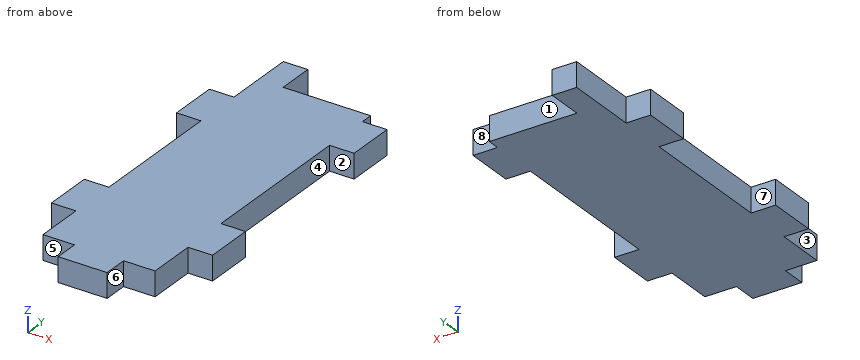
```python
from build123d import *

# Parameters (mm, degrees)
ESQUISSE1_W             = 32.86
ESQUISSE1_H             = 73
BOSS_EXTRU_1_DEPTH      = 5
ESQUISSE2_W             = 5
ESQUISSE2_H             = 33
ESQUISSE2_H_2           = 15
ESQUISSE2_H_3           = 10
ESQUISSE2_H_4           = 28
ENL_V_MAT_EXTRU_1_DEPTH = 5
ESQUISSE3_W             = 10
ESQUISSE3_H             = 5
BOSS_EXTRU_2_DEPTH      = 5


with BuildPart() as part:
    # Esquisse1 → Boss.-Extru.1 (new body)
    with BuildSketch(Plane.XY):
        with Locations((159.387093212, -0.522583191)):
            Rectangle(ESQUISSE1_W, ESQUISSE1_H)
    extrude(amount=BOSS_EXTRU_1_DEPTH)

    # Esquisse2 → Enlèv. mat.-Extru.1 (cut)
    with BuildSketch(Plane.XY.offset(5)):
        Polygon((170.817093212, 25.977416809), (170.817093212, 28.477416809), (152.957093212, 28.477416809), (152.957093212, 35.977416809), (175.817093212, 35.977416809), (175.817093212, 25.977416809), align=None)
        with Locations((173.317093212, -0.522583191)):
            Rectangle(ESQUISSE2_W, ESQUISSE2_H)
        with Locations((145.457093212, 28.477416809)):
            Rectangle(ESQUISSE2_W, ESQUISSE2_H_2)
        with Locations((173.317093212, -32.022583191)):
            Rectangle(ESQUISSE2_W, ESQUISSE2_H_3)
        with Locations((145.457093212, -32.022583191)):
            Rectangle(ESQUISSE2_W, ESQUISSE2_H_3)
        with Locations((145.457093212, -3.022583191)):
            Rectangle(ESQUISSE2_W, ESQUISSE2_H_4)
    extrude(amount=-ENL_V_MAT_EXTRU_1_DEPTH, mode=Mode.SUBTRACT)

    # Esquisse3 → Boss.-Extru.2 (add)
    with BuildSketch(Plane.XY.offset(5)):
        with Locations((159.387093212, -39.522583191)):
            Rectangle(ESQUISSE3_W, ESQUISSE3_H)
    extrude(amount=-BOSS_EXTRU_2_DEPTH)


solid = part.part
```
Model file for the job. Use its own axes, mm. Face numbers are marked on the shaded views. A direction names the side the tool comes from. Round coordinates to 2 decimals unless told otherwise and drop trailing zeros. Loops run counter-clockwise (first coordinate to the right, second up) from the corner with the lowest first, then second, coordinate; pieces in that order, holes last. Notation, with made-up numbers: M 24.25,-14.75 L 81.25,-14.75 A17 cw 81.25,17.25 Z; hole C 13,-39 d3. An arc over 180 degrees is marked long. Put each result on its own line as item: value. Start each with the question number.
Item 1: Cut at D-D (x = 166.5). List the corners of the cut face in (y, z).
Item 2: Drop flat-ended pins along their axis: P1, Ø1.5, axis at x = 144.5, z = 3.5, coming from the -Y side; P2, Ø2.5, axis at x = 174.5, z = 2, coming from the +Y side; P3, Ø8, axis at x = 165, y = 9.5, coming from the -Z side; P4, Ø1.5, axis at x = 146.5, z = 3.5, coming from the +Y side. Give the stop position or say it passes through.
Item 3: Cut at B-B (z = 1.3). List the corners of the cut face in (x, y).
Item 4: Cut at C-C (y = 12). List the corners of the cut face in (x, z), then the cut area to 3 significant figures.
Item 5: Mould opens along Y. For the marked faces 1, 2, 3 and 4 say: released by +Y, released by -Y, zero draft, split by the parting line, or undercut.
Item 6: Drill centre lines: line 1 along Y through (x, z) = (173.5, 2.6); line 2 along Y through (x, z) = (145.5, 0.6); line 3 along Y through (x, z) = (170, 2.65). Where is each one in solid material? Low to high.
Item 7: 3-axis set-ups, long thin cutter, end or side, ignore diameter. For the marked faces 5, 6, 7 and 8: which of +Z, -Z, +X, -X, +Y, -Y reach the whole face in a straight line?
Item 8: Cut at A-A (x = 147). List the corners of the cut face in (y, z).
Answer block:
1. outline: M -37.02,0 L 28.48,0 L 28.48,5 L -37.02,5 Z
2. P1: y = -27.02
2. P2: y = 25.98
2. P3: z = 0
2. P4: y = 20.98
3. outline: M 142.96,-27.02 L 147.96,-27.02 L 147.96,-37.02 L 154.39,-37.02 L 154.39,-42.02 L 164.39,-42.02 L 164.39,-37.02 L 170.82,-37.02 L 170.82,-27.02 L 175.82,-27.02 L 175.82,-17.02 L 170.82,-17.02 L 170.82,15.98 L 175.82,15.98 L 175.82,25.98 L 170.82,25.98 L 170.82,28.48 L 152.96,28.48 L 152.96,35.98 L 147.96,35.98 L 147.96,20.98 L 142.96,20.98 L 142.96,10.98 L 147.96,10.98 L 147.96,-17.02 L 142.96,-17.02 Z
4. outline: M 142.96,0 L 170.82,0 L 170.82,5 L 142.96,5 Z
4. area: 139 mm2
5. face 1: released by +Y
5. face 2: undercut
5. face 3: zero draft
5. face 4: undercut
6. line 1: -27.02 to -17.02, 15.98 to 25.98
6. line 2: -27.02 to -17.02, 10.98 to 20.98
6. line 3: -37.02 to 28.48
7. face 5: +Z, -Z, -X, -Y
7. face 6: +Z, -Z, +X, -Y
7. face 7: +Z, -Z, -X
7. face 8: +Z, -Z, +X, +Y
8. outline: M -27.02,0 L -17.02,0 L -17.02,5 L -27.02,5 Z; M 10.98,0 L 20.98,0 L 20.98,5 L 10.98,5 Z
